Geometry check sheet. Reference: the model listing, model coordinates, mm. Face numbers are marked on the shaded views. Give positions to 0.01 mm unless a question says otherwise; leave off trailing zeros. Write each loop counter-clockwise with the first axis right and the second up, starting at its lowest first coordinate (ties: lowest second). Pieces come first, ordered by that corner, then holes. Notation, with made-up numbers: (51, -24.75) - (95, -24.75) arc R15 ccw to (95, 2.25) - close; hole circle Ø8 at (58, -16). An arc over 180 degrees is marked (long way). Write item = value, one per line. Start each with the question number.
(1) Thickness scan on L1, parallel to Z at x = -3, y = -11.75; L2, parallel to Z at x = -7, y = -22; L3, parallel to X at y = -6, z = -33. Record the ranges inside material, lowest first.
(2) Section check B-B, the plane y = -11. Enter the section's corners in (x, z) (1 decimal).
(3) Section check C-C, the plane z = 32. Enter the section's corners in (x, y), plus the area to 3 significant figures.
(4) Draft check along Z on the marked faces 1, 2, 3 and 4. Enter one of: pulls with the +Z half, pulls with the -Z half, needs draft (parallel to the pull), parting line crosses it, or undercut.
(5) Depth check by flat-ended pin: pin 1 Ø10 at (x, y) = (-7, -5.5) entering from -Z; pin 2 Ø1.5 at (y, z) = (-6, -20) entering from -X; pin 3 Ø5 at (y, z) = (-17.5, -8.5) entering from -X. Enter the tip coordinate at first touch or a pass-through.
(6) Section check D-D, the plane z = -39. Enter the section's corners in (x, y).
(7) Section check A-A, the plane x = 0. Enter the section's corners in (y, z).
```python
from build123d import *

# Parameters (mm, degrees)
F1_DEPTH = 25


with BuildPart() as f1:
    # F0 (on Front) → F1 (new body)
    with BuildSketch(Plane.XZ):
        with BuildLine():
            ThreePointArc((-9.7989449483, 41.9951636275), (0, 50), (9.7989449483, 41.9951636275))
            ThreePointArc((9.7989449483, 41.9951636275), (10.8936502514, 39.1134530116), (11.9093426036, 36.2029539443))
            ThreePointArc((11.9093426036, 36.2029539443), (12.3514530025, 38.0786440394), (12.5, 40))
            ThreePointArc((12.5, 40), (12.2820417112, 42.324102279), (11.6357677755, 44.5671553812))
            ThreePointArc((11.6357677755, 44.5671553812), (0, 52.5), (-11.6357677755, 44.5671553812))
            ThreePointArc((-11.6357677755, 44.5671553812), (-12.493319099, 40.4086292818), (-11.9093426036, 36.2029539443))
            ThreePointArc((-11.9093426036, 36.2029539443), (-10.8936502514, 39.1134530116), (-9.7989449483, 41.9951636275))
        make_face()
        with BuildLine():
            ThreePointArc((9.7989449483, 41.9951636275), (9.9496092758, 41.0026341599), (10, 40))
            ThreePointArc((10, 40), (-1.0026341599, 30.0503907242), (-9.7989449483, 41.9951636275))
            ThreePointArc((-9.7989449483, 41.9951636275), (-10.8936502514, 39.1134530116), (-11.9093426036, 36.2029539443))
            ThreePointArc((-11.9093426036, 36.2029539443), (0, 27.5), (11.9093426036, 36.2029539443))
            ThreePointArc((11.9093426036, 36.2029539443), (10.8936502514, 39.1134530116), (9.7989449483, 41.9951636275))
        make_face()
        with BuildLine():
            ThreePointArc((-11.7644333165, -35.7752977924), (-17.7211555757, 0.20198165), (-11.9093426036, 36.2029539443))
            ThreePointArc((-11.9093426036, 36.2029539443), (-12.493319099, 40.4086292818), (-11.6357677755, 44.5671553812))
            ThreePointArc((-11.6357677755, 44.5671553812), (-20.7751383707, 0.3927164788), (-11.89717505, -43.835000108))
            ThreePointArc((-11.89717505, -43.835000108), (-12.4983050041, -39.7941553412), (-11.7644333165, -35.7752977924))
        make_face()
        with BuildLine():
            ThreePointArc((12.5, -40), (12.3147354104, -37.8558703929), (11.7644333165, -35.7752977924))
            ThreePointArc((11.7644333165, -35.7752977924), (10.8988684939, -38.2401740248), (9.9765535789, -40.6843819744))
            ThreePointArc((9.9765535789, -40.6843819744), (0, -50), (-9.9765535789, -40.6843819744))
            ThreePointArc((-9.9765535789, -40.6843819744), (-10.8988684939, -38.2401740248), (-11.7644333165, -35.7752977924))
            ThreePointArc((-11.7644333165, -35.7752977924), (-12.4983050041, -39.7941553412), (-11.89717505, -43.835000108))
            ThreePointArc((-11.89717505, -43.835000108), (0, -52.5), (11.89717505, -43.835000108))
            ThreePointArc((11.89717505, -43.835000108), (12.3483741465, -41.9410450632), (12.5, -40))
        make_face()
        with BuildLine():
            ThreePointArc((9.9765535789, -40.6843819744), (10.8988684939, -38.2401740248), (11.7644333165, -35.7752977924))
            ThreePointArc((11.7644333165, -35.7752977924), (0, -27.5), (-11.7644333165, -35.7752977924))
            ThreePointArc((-11.7644333165, -35.7752977924), (-10.8988684939, -38.2401740248), (-9.9765535789, -40.6843819744))
            ThreePointArc((-9.9765535789, -40.6843819744), (-0.3423917426, -30.0058633242), (10, -40))
            ThreePointArc((10, -40), (9.9941366758, -40.3423917426), (9.9765535789, -40.6843819744))
        make_face()
        with BuildLine():
            ThreePointArc((12.5, 40), (12.3514530025, 38.0786440394), (11.9093426036, 36.2029539443))
            ThreePointArc((11.9093426036, 36.2029539443), (17.7211555757, 0.20198165), (11.7644333165, -35.7752977924))
            ThreePointArc((11.7644333165, -35.7752977924), (12.3147354104, -37.8558703929), (12.5, -40))
            ThreePointArc((12.5, -40), (12.3483741465, -41.9410450632), (11.89717505, -43.835000108))
            ThreePointArc((11.89717505, -43.835000108), (20.7751383707, 0.3927164788), (11.6357677755, 44.5671553812))
            ThreePointArc((11.6357677755, 44.5671553812), (12.2820417112, 42.324102279), (12.5, 40))
        make_face()
    extrude(amount=F1_DEPTH)


solid = f1.part
```
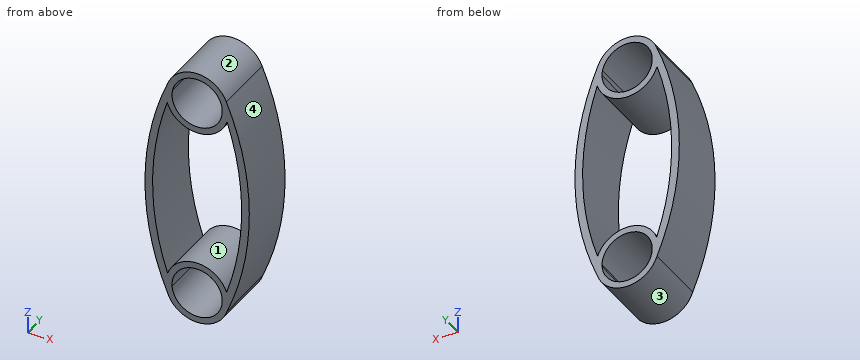
Model answer:
q1.L1 = -52.13 to -49.54, -30.46 to -27.87, 27.87 to 30.46, 49.54 to 52.13
q1.L2 = -50.36 to -47.14, -32.86 to -29.64, 29.64 to 32.86, 47.14 to 50.36
q1.L3 = -15.83 to -12.66, -10.36 to -7.14, 7.14 to 10.36, 12.66 to 15.83
q2.outline = (-11.9, -43.8) arc R12.5 ccw to (11.9, -43.8) arc R112.9 ccw to (11.6, 44.6) arc R12.5 ccw to (-11.6, 44.6) arc R112.9 ccw to start; hole (-11.9, 36.2) arc R113 ccw to (-11.8, -35.8) arc R12.5 cw to (11.8, -35.8) arc R113 ccw to (11.9, 36.2) arc R12.5 cw to start; hole circle Ø20 at (0, -40); hole circle Ø20 at (0, 40)
q3.outline = (-16.16, -25) - (-13.22, -25) - (-13.22, 0) - (-16.16, 0) - close; (-9.6, -25) - (-6, -25) - (-6, 0) - (-9.6, 0) - close; (6, -25) - (9.6, -25) - (9.6, 0) - (6, 0) - close; (13.22, -25) - (16.16, -25) - (16.16, 0) - (13.22, 0) - close
q3.area = 327 mm²
q4.face_1 = undercut
q4.face_2 = pulls with the +Z half
q4.face_3 = pulls with the -Z half
q4.face_4 = parting line crosses it
q5.pin_1 = -52.34
q5.pin_2 = -19.11
q5.pin_3 = -20.61
q6.outline = (-13.81, -25) - (-9.95, -25) - (-9.95, 0) - (-13.81, 0) - close; (9.95, -25) - (13.81, -25) - (13.81, 0) - (9.95, 0) - close
q7.outline = (-25, -52.5) - (0, -52.5) - (0, -50) - (-25, -50) - close; (-25, -30) - (0, -30) - (0, -27.5) - (-25, -27.5) - close; (-25, 27.5) - (0, 27.5) - (0, 30) - (-25, 30) - close; (-25, 50) - (0, 50) - (0, 52.5) - (-25, 52.5) - close
